Could you check a few things on this model? Use its own coordinates, in mm. A direction names the side the tool comes from. Give positions to 0.01 mm unless a question says otherwise; leave off trailing zeros. Order: outer loops, then holes, each group sorted by start corner. A loop starts at its lowest first (then second) coordinate and runs counter-clockwise, first axis right, second up. Notation, with made-up numbers: M 77,5.25 L 127,5.25 A21 cw 127,40.25 Z; hole C 56,25.5 d4. An arc over 180 degrees is marked long. Use a Markdown table: item, result. Add a question column.
```python
from build123d import *

# Parameters (mm, degrees)
F0_R      = 3.4544
F1_DEPTH  = 71.7721196
F3_W      = 4.8468357233
F3_H      = 2.5146
F4_DEPTH  = 39.878
F5_W      = 2.9651967107
F5_H      = 11.1958960486
F6_DEPTH  = 56.642
F8_R      = 3.4544
F8_R_2    = 2.6289
F9_DEPTH  = 58.42
F11_DEPTH = 25.4
F13_DEPTH = 25.4
F15_DEPTH = 25.4


with BuildPart() as f1:
    # F0 (on Front) → F1 (new body)
    with BuildSketch(Plane.XZ):
        Circle(F0_R)
    extrude(amount=F1_DEPTH)

    # F3 (on offset) → F4 (cut)
    with BuildSketch(Plane.XY.offset(25.4)):
        with Locations((3.1854178616, -11.5868196)):
            Rectangle(F3_W, F3_H)
    extrude(amount=-F4_DEPTH, mode=Mode.SUBTRACT)

    # F5 (on offset) → F6 (cut)
    with BuildSketch(Plane.XY.offset(25.4)):
        with Locations((4.0479983554, -5.5979480243)):
            Rectangle(F5_W, F5_H)
    extrude(amount=-F6_DEPTH, mode=Mode.SUBTRACT)

    # F8 (on offset) → F9 (cut)
    with BuildSketch(Plane(origin=(0, -16.9081196, 0), x_dir=(-1, 0, 0), z_dir=(0, 1, 0))):
        Circle(F8_R)
        Circle(F8_R_2, mode=Mode.SUBTRACT)
    extrude(amount=-F9_DEPTH, mode=Mode.SUBTRACT)

    # F10 (on Top) → F11 (cut)
    with BuildSketch(Plane.XY):
        with BuildLine():
            ThreePointArc((5.0546, -41.0381196), (2.1809180413, -42.2284376413), (0.9906, -45.1021196))
            Line((0.9906, -45.1021196), (0.9906, -61.3581196))
            ThreePointArc((0.9906, -61.3581196), (2.1809180413, -64.2318015587), (5.0546, -65.4221196))
            Line((5.0546, -65.4221196), (5.0546, -41.0381196))
        make_face()
        with BuildLine():
            Line((5.0546, -40.7841196), (5.0546, -18.4321196))
            ThreePointArc((5.0546, -18.4321196), (2.1809180413, -19.6224376413), (0.9906, -22.4961196))
            Line((0.9906, -22.4961196), (0.9906, -36.7201196))
            ThreePointArc((0.9906, -36.7201196), (2.1809180413, -39.5938015587), (5.0546, -40.7841196))
        make_face()
    extrude(amount=F11_DEPTH, mode=Mode.SUBTRACT)

    # F12 (on face) → F13 (cut)
    with BuildSketch(Plane.XY):
        with BuildLine():
            ThreePointArc((2.6289, -41.8414332443), (1.4231993887, -43.2775578444), (0.9906, -45.1021196))
            Line((0.9906, -45.1021196), (0.9906, -61.3581196))
            ThreePointArc((0.9906, -61.3581196), (1.4231993887, -63.1826813556), (2.6289, -64.6188059557))
            Line((2.6289, -64.6188059557), (2.6289, -41.8414332443))
        make_face()
    extrude(amount=-F13_DEPTH, mode=Mode.SUBTRACT)

    # F14 (on face) → F15 (cut)
    with BuildSketch(Plane.XY):
        with BuildLine():
            ThreePointArc((2.6289, -19.2354332443), (1.4231993887, -20.6715578444), (0.9906, -22.4961196))
            Line((0.9906, -22.4961196), (0.9906, -36.7201196))
            ThreePointArc((0.9906, -36.7201196), (1.4231993887, -38.5446813556), (2.6289, -39.9808059557))
            Line((2.6289, -39.9808059557), (2.6289, -19.2354332443))
        make_face()
    extrude(amount=-F15_DEPTH, mode=Mode.SUBTRACT)


solid = f1.part
```
1) Please list where these lines run through material, in increasing order: line 1 (Y direction, x = 1.75, z = 2.5); line 2 (Y direction, x = 2, z = 0.75); line 3 (Y direction, x = -2.75, z = 1.75). Write a range as from..to.
2) For pin 1 (4 mm diameter, centred on y = -30, z = 1, fed in from +X); pin 2 (2 mm diameter, centred on y = -21.5, z = -2, fed in from -X); pin 3 (2 mm diameter, centred on y = -12, z = 1, fed in from +X), each with a flat end and sliding along its axis, tell me the tip position at first contact or that it passes through.
3) Suppose I cut it at A-A on x = 0. Please give me the cut outline in (y, z), and give its area (3 significant figures).
4) Suppose I cut it at B-B on y = -23.5. Please give me the cut outline in (x, z), and give its area (3 significant figures).
5) Suppose I cut it at C-C on z = -1. Please give me the cut outline in (x, y), and give its area (3 significant figures).
6) We'd pull the mould along Y, two halves only. Please class faces 1 (the face through (0.762, -12, 0)), 2 (the face through (0, 0, 0)), 3 (the face through (1, -16.908, -3)), 4 (the face through (0.991, -53, 0)): pulls with the +Y half, pulls with the -Y half, needs draft (parallel to the pull), parting line crosses it, or undercut.
7) For faces 5 (the face through (-2.508, -43.956, 0.79)), 6 (the face through (2.565, -5, 0)), 7 (the face through (0.991, -30, 0)), 8 (the face through (0, -71.772, 0)), which set-ups out of +Z, -Z, +X, -X, +Y, -Y let a thin tool reach every point of the face, with its end or its side?
Values found:
| question | item | result |
|---|---|---|
| 1 | line 1 | y = -16.91..-12.84, -10.33..0 |
| 1 | line 2 | y = -71.77..-64.04, -42.42..-39.4, -19.82..-12.84, -10.33..0 |
| 1 | line 3 | y = -16.91..0 |
| 2 | pin 1 | stops at x = 0.99 |
| 2 | pin 2 | stops at x = -2.43 |
| 2 | pin 3 | stops at x = 3.42 |
| 3 | outline | M -71.77,-2.63 L -16.91,-2.63 L -16.91,-3.45 L 0,-3.45 L 0,3.45 L -16.91,3.45 L -16.91,2.63 L -71.77,2.63 Z |
| 3 | area | 405 mm^2 |
| 4 | outline | M 0.99,-2.44 L 0.99,2.44 A2.63 ccw long Z |
| 4 | area | 15.9 mm^2 |
| 5 | outline | M -3.31,-16.91 L -2.43,-16.91 L -2.43,-71.77 L 2.43,-71.77 L 2.43,-64.46 A4.06 cw 0.99,-61.36 L 0.99,-45.1 A4.06 cw 2.43,-42 L 2.43,-39.82 A4.06 cw 0.99,-36.72 L 0.99,-22.5 A4.06 cw 2.43,-19.39 L 2.43,-16.91 L 3.31,-16.91 L 3.31,-12.84 L 0.76,-12.84 L 0.76,-10.33 L 2.57,-10.33 L 2.57,0 L -3.31,0 Z |
| 5 | area | 308 mm^2 |
| 6 | face 1 | undercut |
| 6 | face 2 | pulls with the +Y half |
| 6 | face 3 | pulls with the -Y half |
| 6 | face 4 | undercut |
| 7 | face 5 | -Y |
| 7 | face 6 | +Z, -Z, +X, +Y |
| 7 | face 7 | +Z, -Z, +X |
| 7 | face 8 | +Z, -Z, +X, -X, -Y |
